Could you check a few things on this model? Use its own coordinates, in mm. A direction names the side the tool comes from. Coordinates: 2 decimals unless noted, no trailing zeros. Loops run counter-clockwise (first coordinate to the right, second up) from the corner with the lowest first, then second, coordinate; pieces in that order, holes last.
from build123d import *

# Parameters (mm, degrees)
F0_W     = 63.5
F0_H     = 101.6
F1_DEPTH = 31.75
F2_W     = 53.975
F2_H     = 88.9
F3_DEPTH = 57.15
F4_W     = 53.975
F4_H     = 1.27
F5_DEPTH = 28.575


with BuildPart() as f1:
    # F0 (on Front) → F1 (new body, symmetric)
    with BuildSketch(Plane.XZ):
        Rectangle(F0_W, F0_H)
    extrude(amount=F1_DEPTH, both=True)

    # F2 (on face) → F3 (cut)
    with BuildSketch(Plane.XZ.offset(31.75)):
        Rectangle(F2_W, F2_H)
    extrude(amount=-F3_DEPTH, mode=Mode.SUBTRACT)

    # F4 (on Front) → F5 (join, symmetric)
    with BuildSketch(Plane.XZ):
        with Locations((-0.089094, 18.991973)):
            Rectangle(F4_W, F4_H)
        with Locations((0, -14.710611)):
            Rectangle(F4_W, F4_H)
    extrude(amount=F5_DEPTH, both=True)


solid = f1.part
1) Imagine slicing it at B-B on z = 22. List the corners of the cut face in (x, y) for me, plus the area to 3 significant figures.
2) If I drill on L1, parallel to Z at x = 16.5, y = 1; L2, parallel to X at y = 12, z = -30; L3, parallel to Y at x = 21.5, z = 8.5, over which ranges is the centre line in solid material (lowest first)?
3) We'd pull the mould along X, two halves only. Please class faces 1 (the flat face through (-31.75, 0, -1)), 2 (the flat face through (0, -4, -44.45)), 3 (the flat face through (31.75, 0, -1)): released by +X, released by -X, zero draft, split by the parting line, or undercut.
4) Imagine slicing it at A-A on y = 8. List the corners of the cut face in (x, z) for me.
5) For faces 4 (the flat face through (0, 0, -50.8)), 5 (the flat face through (-26.988, -4, -1)), which set-ups out of +Z, -Z, +X, -X, +Y, -Y let a thin tool reach every point of the face, with its end or its side?
6) Will these pins go through, and if not, where does the flat tip stop? pin 1 (4 mm diameter, centred on x = 8, z = 28.5, fed in from -Y); pin 2 (1.4 mm diameter, centred on x = -2, z = 19, fed in from -Y) (3 decimals).
7) Imagine slicing it at C-C on x = -22.5. List the corners of the cut face in (y, z) for me (3 decimals), plus the area to 3 significant figures.
Solved:
1. outline: (-31.75, -31.75) - (-26.99, -31.75) - (-26.99, 25.4) - (26.99, 25.4) - (26.99, -31.75) - (31.75, -31.75) - (31.75, 31.75) - (-31.75, 31.75) - close
1. area: 948 mm2
2. L1: z = -50.8 to -44.45, -15.35 to -14.08, 18.36 to 19.63, 44.45 to 50.8
2. L2: x = -31.75 to -26.99, 26.99 to 31.75
2. L3: y = 25.4 to 31.75
3. face 1: released by -X
3. face 2: undercut
3. face 3: released by +X
4. outline: (-31.75, -50.8) - (31.75, -50.8) - (31.75, 50.8) - (-31.75, 50.8) - close; hole (-26.99, -44.45) - (26.99, -44.45) - (26.99, -15.35) - (-26.99, -15.35) - close; hole (-26.99, -14.08) - (26.99, -14.08) - (26.99, 44.45) - (-26.99, 44.45) - (-26.99, 19.63) - (26.9, 19.63) - (26.9, 18.36) - (-26.99, 18.36) - close
5. face 4: -Z, +X, -X, +Y, -Y
5. face 5: -Y
6. pin 1: stops at y = 25.4
6. pin 2: stops at y = -28.575
7. outline: (-31.75, -50.8) - (31.75, -50.8) - (31.75, 50.8) - (-31.75, 50.8) - (-31.75, 44.45) - (25.4, 44.45) - (25.4, 19.627) - (-28.575, 19.627) - (-28.575, 18.357) - (25.4, 18.357) - (25.4, -14.076) - (-28.575, -14.076) - (-28.575, -15.346) - (25.4, -15.346) - (25.4, -44.45) - (-31.75, -44.45) - close
7. area: 1,510 mm2
